Could you check a few things on this model? Use its own coordinates, in mm. A direction names the side the tool comes from. Coordinates: 2 decimals unless noted, no trailing zeros. Loops run counter-clockwise (first coordinate to the right, second up) from the corner with the lowest first, then second, coordinate; pieces in that order, holes last. Notation, with made-up numbers: (19.25, 83.5) -> (46.25, 83.5) arc R33 cw to (46.25, 111.5) -> close; hole circle Ø2 at (56.5, 69). An arc over 180 degrees is marked (long way). One line per question, with ' | ' between items.
from build123d import *

# Parameters (mm, degrees)
CROQUIS1_R                 = 60.239614391
CROQUIS1_R_2               = 18.75
CROQUIS1_R_3               = 4
SALIENTE_EXTRUIR1_DEPTH    = 10
CROQUIS2_R                 = 40
CROQUIS2_R_2               = 18.75
SALIENTE_EXTRUIR2_DEPTH    = 25
CHAFL_N2_SIZE              = 0.5
REDONDEO1_R                = 0.5
CORTAR_EXTRUIR1_DEPTH      = 93.101152457
CORTAR_EXTRUIR1_DEPTH_BACK = 93.101152457
CROQUIS3_R                 = 4.7625


with BuildPart() as part:
    # Croquis1 → Saliente-Extruir1 (new body)
    with BuildSketch(Plane(origin=(0, 0, 0), x_dir=(1, 0, 0), z_dir=(0, 1, 0))):
        with Locations(Location((0, 0, 0), (0, 0, 270))):
            Circle(CROQUIS1_R)
        with Locations(Location((0, 0, 0), (0, 0, 270))):
            Circle(CROQUIS1_R_2, mode=Mode.SUBTRACT)
        with Locations(Location((25, -43.301270189, 0), (0, 0, 270))):
            Circle(CROQUIS1_R_3, mode=Mode.SUBTRACT)
        with Locations(Location((-25, -43.301270189, 0), (0, 0, 270))):
            Circle(CROQUIS1_R_3, mode=Mode.SUBTRACT)
        with Locations(Location((-50, 0, 0), (0, 0, 270))):
            Circle(CROQUIS1_R_3, mode=Mode.SUBTRACT)
        with Locations(Location((-25, 43.301270189, 0), (0, 0, 270))):
            Circle(CROQUIS1_R_3, mode=Mode.SUBTRACT)
        with Locations(Location((25, 43.301270189, 0), (0, 0, 270))):
            Circle(CROQUIS1_R_3, mode=Mode.SUBTRACT)
        with Locations(Location((50, 0, 0), (0, 0, 270))):
            Circle(CROQUIS1_R_3, mode=Mode.SUBTRACT)
    extrude(amount=SALIENTE_EXTRUIR1_DEPTH)

    # Croquis2 → Saliente-Extruir2 (add)
    with BuildSketch(Plane(origin=(0, 10, 0), x_dir=(1, 0, 0), z_dir=(0, 1, 0))):
        with Locations(Location((0, 0, 0), (0, 0, 270))):
            Circle(CROQUIS2_R)
        with Locations(Location((0, 0, 0), (0, 0, 270))):
            Circle(CROQUIS2_R_2, mode=Mode.SUBTRACT)
    extrude(amount=SALIENTE_EXTRUIR2_DEPTH)

    # Chaflán2
    chafl_n2_edges = [part.edges().sort_by_distance(p)[0] for p in [
        (0, 0, -60.239614391),
        (0, 35, -40),
        (0, 35, -18.75),
        (0, 10, -60.239614391),
    ]]
    chamfer(chafl_n2_edges, length=CHAFL_N2_SIZE)

    # Redondeo1
    redondeo1_edges = [part.edges().sort_by_distance(p)[0] for p in [
        (0, 10, -40),
    ]]
    fillet(redondeo1_edges, radius=REDONDEO1_R)

    # Croquis3 → Cortar-Extruir1 (cut, two sides: drawn at the far end of the back side and taken through both)
    with BuildSketch(Plane(origin=(0, 0, 0), x_dir=(0, 0, -1), z_dir=(1, 0, 0)).offset(-CORTAR_EXTRUIR1_DEPTH_BACK)):
        with Locations((0, 22.5)):
            Circle(CROQUIS3_R)
    extrude(amount=CORTAR_EXTRUIR1_DEPTH + CORTAR_EXTRUIR1_DEPTH_BACK, mode=Mode.SUBTRACT)


solid = part.part
1) On a 3-axis mill with a long thin cutter (end or side, diameter ignored), from which of +Z, -Z, +X, -X, +Y, -Y can I reach the whole of each face in a straight line? I mean faces 5 (the face through (-52.4, 4.9, -3.2)), 6 (the face through (-12, 10, 39)). Say none if no direction works.
Data:
face 5: +Y, -Y | face 6: +Y
2) I'm going to push flat-ended pins straight in: pin 1 Ø8 at (x, y) = (-18, 17) entering from -Z; pin 2 Ø9 at (x, z) = (-25, 43.3) entering from -Y; pin 3 Ø9 at (x, z) = (-50, 0) entering from +Y; pin 4 Ø4 at (y, z) = (21, 39) entering from +X. Where does each tip first touch, or does it pass through?
Data:
pin 1: z = -37.47 | pin 2: y = 0 | pin 3: y = 10 | pin 4: x = 15.2
3) I need wall thicknesses on line 1 along X through (y, z) = (8.25, 0); line 2 along Y through (x, z) = (-35, 0); line 3 along Y through (x, z) = (-5, -42). Which ranges of each line are inside material? Lowest first, please. Write a range as from..to.
Data:
line 1: -60.24..-54, -46..-18.75, 18.75..46, 54..60.24 | line 2: 0..17.74, 27.26..35 | line 3: 0..10
4) If we section it at B-B on y = 20.5: Please give me the cut outline in (x, z).
Data:
outline: (-39.77, -4.32) arc R40 ccw to (39.77, -4.32) -> (18.25, -4.32) arc R18.75 cw to (-18.25, -4.32) -> close; (-39.77, 4.32) -> (-18.25, 4.32) arc R18.75 cw to (18.25, 4.32) -> (39.77, 4.32) arc R40 ccw to start
5) We'd pull the mould along Y, two halves only. Please class faces 1 (the face through (28.91, 17.85, 1.03)), 2 (the face through (14, 0, -14)), 3 (the face through (-29.21, 17.85, 1.03)), 4 (the face through (26.201, 4.93, 47.117)): pulls with the +Y half, pulls with the -Y half, needs draft (parallel to the pull), parting line crosses it, or undercut.
Data:
face 1: undercut | face 2: pulls with the -Y half | face 3: undercut | face 4: needs draft
6) If we section it at A-A on y = 3.5: Please give me the cut outline in (x, z).
Data:
outline: circle Ø120.48 at (0, 0); hole circle Ø8 at (-50, 0); hole circle Ø8 at (-25, -43.3); hole circle Ø8 at (-25, 43.3); hole circle Ø37.5 at (0, 0); hole circle Ø8 at (25, -43.3); hole circle Ø8 at (25, 43.3); hole circle Ø8 at (50, 0)
7) If we section it at C-C on x = -25: Give the number of separate pieces and of enclosed holes in the cut face, and give its area (3 significant figures).
Data:
separate pieces: 3 | enclosed holes: 1 | area: 2,430 mm²
